from build123d import *

# Parameters (mm, degrees)
SKETCH1_W                                 = 152.4
SKETCH1_H                                 = 76.2
BOSS_EXTRUDE1_DEPTH                       = 25.4
SKETCH2_OUTSIDE_W                         = 188.854
SKETCH2_OUTSIDE_H                         = 112.654
CUT_EXTRUDE1_DEPTH                        = 6.35
CUT_EXTRUDE3_DEPTH                        = 10.3124
BOSS_EXTRUDE3_DEPTH                       = 5.1562
SKETCH11_R                                = 1.9812
BOSS_EXTRUDE4_DEPTH                       = 2.3622
SKETCH12_R                                = 1.9812
BOSS_EXTRUDE5_DEPTH                       = 7.1374
SKETCH9_W                                 = 1.984375
SKETCH9_H                                 = 20.2438
F_5_32_0_15625_DIAMETER_HOLE1_AT_2_COUNT  = 2
F_5_32_0_15625_DIAMETER_HOLE1_AT_2_PITCH  = 9.865104057
F_5_32_0_15625_DIAMETER_HOLE1_AT_3_COUNT  = 2
F_5_32_0_15625_DIAMETER_HOLE1_AT_3_PITCH  = 24.013204868
F_5_32_0_15625_DIAMETER_HOLE1_AT_4_COUNT  = 2
F_5_32_0_15625_DIAMETER_HOLE1_AT_4_PITCH  = 29.953363952
F_5_32_0_15625_DIAMETER_HOLE1_AT_5_COUNT  = 2
F_5_32_0_15625_DIAMETER_HOLE1_AT_5_PITCH  = 33.9598
F_5_32_0_15625_DIAMETER_HOLE1_AT_6_COUNT  = 2
F_5_32_0_15625_DIAMETER_HOLE1_AT_6_PITCH  = 32.495349482
F_5_32_0_15625_DIAMETER_HOLE1_AT_7_COUNT  = 2
F_5_32_0_15625_DIAMETER_HOLE1_AT_7_PITCH  = 24.013204868
F_5_32_0_15625_DIAMETER_HOLE1_AT_8_COUNT  = 2
F_5_32_0_15625_DIAMETER_HOLE1_AT_8_PITCH  = 16.002
F_5_32_0_15625_DIAMETER_HOLE1_AT_9_COUNT  = 2
F_5_32_0_15625_DIAMETER_HOLE1_AT_9_PITCH  = 25.499228315
F_5_32_0_15625_DIAMETER_HOLE1_AT_10_COUNT = 2
F_5_32_0_15625_DIAMETER_HOLE1_AT_10_PITCH = 62.467521


with BuildPart() as part:
    # Sketch1 → Boss-Extrude1 (new body)
    with BuildSketch(Plane.XY):
        Rectangle(SKETCH1_W, SKETCH1_H)
    extrude(amount=BOSS_EXTRUDE1_DEPTH)

    # Sketch2 outside → Cut-Extrude1 (cut)
    with BuildSketch(Plane.XY.offset(25.4)):
        Rectangle(SKETCH2_OUTSIDE_W, SKETCH2_OUTSIDE_H)
        with BuildLine():
            Line((-71.4248, 38.1), (76.2, 38.1))
            Line((76.2, 38.1), (76.2, -33.3248))
            Line((76.2, -33.3248), (-65.0748, -33.3248))
            ThreePointArc((-65.0748, -33.3248), (-69.564928061, -31.464928061), (-71.4248, -26.9748))
            Line((-71.4248, -26.9748), (-71.4248, 38.1))
        make_face(mode=Mode.SUBTRACT)
    extrude(amount=-CUT_EXTRUDE1_DEPTH, mode=Mode.SUBTRACT)

    # Sketch5 → Cut-Extrude3 (cut)
    with BuildSketch(Plane.XY.offset(25.4)):
        with BuildLine():
            Line((-53.34, 28.575), (62.7126, 28.575))
            ThreePointArc((62.7126, 28.575), (67.75950394, 26.48450394), (69.85, 21.4376))
            Line((69.85, 21.4376), (69.85, -15.769127551))
            ThreePointArc((69.85, -15.769127551), (68.078781442, -20.475142372), (63.644217644, -22.845466105))
            Line((63.644217644, -22.845466105), (0, -31.224386314))
            Line((0, -31.224386314), (-56.411435655, -23.797679918))
            ThreePointArc((-56.411435655, -23.797679918), (-61.142298141, -21.066315188), (-62.556156564, -15.78972372))
            Line((-62.556156564, -15.78972372), (-60.4774, 0))
            Line((-60.4774, 0), (-60.4774, 21.4376))
            ThreePointArc((-60.4774, 21.4376), (-58.38690394, 26.48450394), (-53.34, 28.575))
        make_face()
    extrude(amount=-CUT_EXTRUDE3_DEPTH, mode=Mode.SUBTRACT)

    # Sketch6 → Boss-Extrude3 (add)
    with BuildSketch(Plane.XY.offset(15.0876)):
        with BuildLine():
            ThreePointArc((-20.500992736, 6.223796015), (-21.4249, 0), (-20.500992736, -6.223796015))
            ThreePointArc((-20.500992736, -6.223796015), (-14.956430755, -9.185870024), (-11.994356746, -3.641308042))
            ThreePointArc((-11.994356746, -3.641308042), (-12.5349, 0), (-11.994356746, 3.641308042))
            ThreePointArc((-11.994356746, 3.641308042), (-14.956430755, 9.185870024), (-20.500992736, 6.223796015))
        make_face()
        with BuildLine():
            ThreePointArc((20.500992736, -6.223796015), (21.4249, 0), (20.500992736, 6.223796015))
            ThreePointArc((20.500992736, 6.223796015), (14.956430755, 9.185870024), (11.994356746, 3.641308042))
            ThreePointArc((11.994356746, 3.641308042), (12.5349, 0), (11.994356746, -3.641308042))
            ThreePointArc((11.994356746, -3.641308042), (14.956430755, -9.185870024), (20.500992736, -6.223796015))
        make_face()
        with BuildLine():
            ThreePointArc((-6.223796015, -20.500992736), (0, -21.4249), (6.223796015, -20.500992736))
            ThreePointArc((6.223796015, -20.500992736), (9.185870024, -14.956430755), (3.641308042, -11.994356746))
            ThreePointArc((3.641308042, -11.994356746), (0, -12.5349), (-3.641308042, -11.994356746))
            ThreePointArc((-3.641308042, -11.994356746), (-9.185870024, -14.956430755), (-6.223796015, -20.500992736))
        make_face()
        with BuildLine():
            ThreePointArc((6.223796015, 20.500992736), (0, 21.4249), (-6.223796015, 20.500992736))
            ThreePointArc((-6.223796015, 20.500992736), (-9.185870024, 14.956430755), (-3.641308042, 11.994356746))
            ThreePointArc((-3.641308042, 11.994356746), (0, 12.5349), (3.641308042, 11.994356746))
            ThreePointArc((3.641308042, 11.994356746), (9.185870024, 14.956430755), (6.223796015, 20.500992736))
        make_face()
    extrude(amount=BOSS_EXTRUDE3_DEPTH)

    # Sketch11 → Boss-Extrude4 (add)
    with BuildSketch(Plane.XY.offset(15.0876)):
        Polygon((-38.90278116, 8.902536881), (-47.755912042, 6.530347611), (-50.128101312, -2.32278327), (-43.647159701, -8.803724881), (-34.794028819, -6.431535611), (-32.421839549, 2.42159527), align=None)
        with Locations((-41.274970431, 0.049406)):
            Circle(SKETCH11_R, mode=Mode.SUBTRACT)
    extrude(amount=BOSS_EXTRUDE4_DEPTH)

    # Sketch12 → Boss-Extrude5 (add)
    with BuildSketch(Plane.XY.offset(15.0876)):
        with BuildLine():
            Line((52.743870809, -12.545946722), (60.112191116, -2.022894761))
            ThreePointArc((60.112191116, -2.022894761), (60.390997888, -1.256879453), (60.24944398, -0.454087351))
            Line((60.24944398, -0.454087351), (54.820373811, 11.188591199))
            ThreePointArc((54.820373811, 11.188591199), (54.29638848, 11.8130526), (53.530373171, 12.091859371))
            Line((53.530373171, 12.091859371), (40.732982694, 13.21148596))
            ThreePointArc((40.732982694, 13.21148596), (39.930190592, 13.069932053), (39.305729191, 12.545946722))
            Line((39.305729191, 12.545946722), (31.937408884, 2.022894761))
            ThreePointArc((31.937408884, 2.022894761), (31.658602112, 1.256879453), (31.80015602, 0.454087351))
            Line((31.80015602, 0.454087351), (37.229226189, -11.188591199))
            ThreePointArc((37.229226189, -11.188591199), (37.75321152, -11.8130526), (38.519226829, -12.091859371))
            Line((38.519226829, -12.091859371), (51.316617306, -13.21148596))
            ThreePointArc((51.316617306, -13.21148596), (52.119409408, -13.069932053), (52.743870809, -12.545946722))
        make_face()
        with Locations((46.0248, 0)):
            Circle(SKETCH12_R, mode=Mode.SUBTRACT)
    extrude(amount=BOSS_EXTRUDE5_DEPTH)

    # Sketch9 → 5/32 (0.15625) Diameter Hole1 (revolve, cut)
    with BuildSketch(Plane(origin=(-16.247674741, 4.932552029, 20.2438), x_dir=(0, -1, 0), z_dir=(1, 0, 0))):
        with Locations((0.9921875, 10.1219)):
            Rectangle(SKETCH9_W, SKETCH9_H)
    f_5_32_0_15625_diameter_hole1 = revolve(axis=Axis((-16.247674741, 4.932552029, 26.5938), (0, 0, -1)), mode=Mode.SUBTRACT)

    # 5/32 (0.15625) Diameter Hole1 at 2: 5/32 (0.15625) Diameter Hole1 ×2
    with Locations(*[(0, -i * F_5_32_0_15625_DIAMETER_HOLE1_AT_2_PITCH, 0) for i in range(1, F_5_32_0_15625_DIAMETER_HOLE1_AT_2_COUNT)]):
        add(f_5_32_0_15625_diameter_hole1, mode=Mode.SUBTRACT)

    # 5/32 (0.15625) Diameter Hole1 at 3: 5/32 (0.15625) Diameter Hole1 ×2
    with Locations(*[Vector(0.471204188, -0.882024157, 0) * (i * F_5_32_0_15625_DIAMETER_HOLE1_AT_3_PITCH) for i in range(1, F_5_32_0_15625_DIAMETER_HOLE1_AT_3_COUNT)]):
        add(f_5_32_0_15625_diameter_hole1, mode=Mode.SUBTRACT)

    # 5/32 (0.15625) Diameter Hole1 at 4: 5/32 (0.15625) Diameter Hole1 ×2
    with Locations(*[Vector(0.707106781, -0.707106781, 0) * (i * F_5_32_0_15625_DIAMETER_HOLE1_AT_4_PITCH) for i in range(1, F_5_32_0_15625_DIAMETER_HOLE1_AT_4_COUNT)]):
        add(f_5_32_0_15625_diameter_hole1, mode=Mode.SUBTRACT)

    # 5/32 (0.15625) Diameter Hole1 at 5: 5/32 (0.15625) Diameter Hole1 ×2
    with Locations(*[Vector(0.956876939, -0.290493585, 0) * (i * F_5_32_0_15625_DIAMETER_HOLE1_AT_5_PITCH) for i in range(1, F_5_32_0_15625_DIAMETER_HOLE1_AT_5_COUNT)]):
        add(f_5_32_0_15625_diameter_hole1, mode=Mode.SUBTRACT)

    # 5/32 (0.15625) Diameter Hole1 at 6: 5/32 (0.15625) Diameter Hole1 ×2
    with Locations(*[(i * F_5_32_0_15625_DIAMETER_HOLE1_AT_6_PITCH, 0, 0) for i in range(1, F_5_32_0_15625_DIAMETER_HOLE1_AT_6_COUNT)]):
        add(f_5_32_0_15625_diameter_hole1, mode=Mode.SUBTRACT)

    # 5/32 (0.15625) Diameter Hole1 at 7: 5/32 (0.15625) Diameter Hole1 ×2
    with Locations(*[Vector(0.882024157, 0.471204188, 0) * (i * F_5_32_0_15625_DIAMETER_HOLE1_AT_7_PITCH) for i in range(1, F_5_32_0_15625_DIAMETER_HOLE1_AT_7_COUNT)]):
        add(f_5_32_0_15625_diameter_hole1, mode=Mode.SUBTRACT)

    # 5/32 (0.15625) Diameter Hole1 at 8: 5/32 (0.15625) Diameter Hole1 ×2
    with Locations(*[Vector(0.707106781, 0.707106781, 0) * (i * F_5_32_0_15625_DIAMETER_HOLE1_AT_8_PITCH) for i in range(1, F_5_32_0_15625_DIAMETER_HOLE1_AT_8_COUNT)]):
        add(f_5_32_0_15625_diameter_hole1, mode=Mode.SUBTRACT)

    # 5/32 (0.15625) Diameter Hole1 at 9: 5/32 (0.15625) Diameter Hole1 ×2
    with Locations(*[Vector(-0.981492278, -0.191501718, 0) * (i * F_5_32_0_15625_DIAMETER_HOLE1_AT_9_PITCH) for i in range(1, F_5_32_0_15625_DIAMETER_HOLE1_AT_9_COUNT)]):
        add(f_5_32_0_15625_diameter_hole1, mode=Mode.SUBTRACT)

    # 5/32 (0.15625) Diameter Hole1 at 10: 5/32 (0.15625) Diameter Hole1 ×2
    with Locations(*[Vector(0.996877637, -0.078961866, 0) * (i * F_5_32_0_15625_DIAMETER_HOLE1_AT_10_PITCH) for i in range(1, F_5_32_0_15625_DIAMETER_HOLE1_AT_10_COUNT)]):
        add(f_5_32_0_15625_diameter_hole1, mode=Mode.SUBTRACT)


solid = part.part
Check sheet for the modelled part. Datum: model origin and axes. Units: mm. A direction names the side the tool comes from. Give positions to 0.01 mm unless a question says otherwise; leave off trailing zeros. Loops run counter-clockwise (first coordinate to the right, second up) from the corner with the lowest first, then second, coordinate; pieces in that order, holes last. Notation, with made-up numbers: M 83.5,-9 L 105.5,-9 A10 cw 105.5,1 Z; hole C 14.25,25.5 d6. An arc over 180 degrees is marked long. Return JSON: item names as keys, results as strings. Group by question number.
1. Mould release check, pull along X, two halves, no side actions. Record for faces 1 (the cylindrical face through (-69.52, -31.51, 22.27)), 2 (the flat face through (-46.93, -5.52, 16.25)), 3 (the flat face through (-1, 38.1, 13)): released by +X, released by -X, zero draft, split by the parting line, or undercut.
2. Tool access check on faces 4 (the cylindrical face through (-5.02, 18.23, 9.98)), 5 (the flat face through (32.268, -26.976, 20.316)), 6 (the flat face through (-71.425, 5, 22)). Record the directions out of +Z, -Z, +X, -X, +Y, -Y that give a thin tool (end or side, any length) a straight path to the whole face; none if there is none.
3. Go/stop test with flat-tipped pins: pin 1 (10.5 mm diameter, centred on x = -4.5, y = -18, fed in from +Z); pin 2 (8 mm diameter, centred on x = -32, y = 3, fed in from +Z); pin 3 (3 mm diameter, centred on x = 57, y = -16, fed in from +Z); pin 4 (3 mm diameter, centred on x = -16.25, y = 4.93, fed in from +Z). Record where each tip stops, or that it passes through.
4. Cross-section at A-A on x = -37. Record the boundary of the cut face in (y, z) (3 decimals), plus the area to 3 significant figures.
5. Thickness scan on L1, parallel to X at y = 0, z = 15; L2, parallel to X at y = 0, z = 20.7; L3, parallel to X at y = 20, z = 15.75. Record the ranges inside material, lowest first.
Return value:
{
 "1": {"face 1": "released by -X", "face 2": "undercut", "face 3": "zero draft"},
 "2": {"face 4": "+Z, -Z", "face 5": "+Z", "face 6": "+Z, -X, +Y, -Y"},
 "3": {"pin 1": "z = 20.24", "pin 2": "z = 17.45", "pin 3": "z = 15.09", "pin 4": "through"},
 "4": {"outline": "M -38.1,0 L 38.1,0 L 38.1,25.4 L 28.575,25.4 L 28.575,15.088 L 7,15.088 L 7,17.45 L -7.023,17.45 L -7.023,15.088 L -26.353,15.088 L -26.353,25.4 L -33.325,25.4 L -33.325,19.05 L -38.1,19.05 Z", "area": "1,370 mm^2"},
 "5": {"L1": "-76.2 to -43.26, -39.29 to 44.04, 48.01 to 76.2", "L2": "-71.42 to -60.48, 32.01 to 44.04, 48.01 to 60.04, 69.85 to 76.2", "L3": "-76.2 to -60.48, -7.32 to 7.32, 69.85 to 76.2"}
}
